Input: part model. Units: mm. Frame: model coordinates. A direction names the side the tool comes from. Give positions to 0.01 mm unless a question says otherwise; leave off trailing zeros. Write each loop counter-clockwise with the first axis right and the second up, starting at its lowest first coordinate (ties: lowest second). Pieces come first, ordered by that corner, then holes.
```python
from build123d import *

# Parameters (mm, degrees)
CROQUIS1_W              = 360
CROQUIS1_H              = 187
SALIENTE_EXTRUIR1_DEPTH = 80
VACIADO1_T              = -4
CORTAR_EXTRUIR1_DEPTH   = 361


with BuildPart() as part:
    # Croquis1 → Saliente-Extruir1 (new body)
    with BuildSketch(Plane(origin=(0, 0, 0), x_dir=(1, 0, 0), z_dir=(0, 1, 0))):
        Rectangle(CROQUIS1_W, CROQUIS1_H)
    extrude(amount=SALIENTE_EXTRUIR1_DEPTH)

    # Vaciado1
    vaciado1_openings = [part.faces().sort_by_distance(p)[0] for p in [
        (0, 80, 0),
    ]]
    offset(amount=VACIADO1_T, openings=vaciado1_openings, kind=Kind.INTERSECTION)

    # Croquis2 → Cortar-Extruir1 (cut, through all)
    with BuildSketch(Plane.ZY.offset(180)):
        Polygon((-93.5, 80), (93.5, 40), (93.5, 80), align=None)
    extrude(amount=-CORTAR_EXTRUIR1_DEPTH, mode=Mode.SUBTRACT)


solid = part.part
```
Item 1: Ray query, line 1 (X direction, y = 54, z = 12); line 2 (Z direction, x = 82, y = 24); line 3 (Y direction, x = -21, z = -2). Return the intervals inside material, ascending.
Item 2: Pin query (flat end, axial travel): pin 1 (10 mm diameter, centred on x = 22, z = 22, fed in from -Y); pin 2 (2 mm diameter, centred on x = 104.5, z = -65.5, fed in from +Y). Return the tip coordinate at first contact, or that it passes through.
Item 3: Section B-B (x = 78). Return loops of the section in (y, z), and give its area (3 significant figures).
Item 4: Section A-A (y = 34). Return loops of the section in (x, z).
Item 5: Mould query, pull axis Z, two halves, no side actions, for faces 1 (the flat face through (-0.84, 79.35, -90.47)), 2 (the flat face through (-2, 41, -89.5)), 3 (the flat face through (180, 31, 1)), 4 (the flat face through (-3, 39, -93.5)). Classes: +Z half, -Z half, draft (parallel to the pull), parting line (faces both ways), or undercut.
Item 6: Section C-C (y = 58). Return loops of the section in (x, z), and give its area (3 significant figures).
Item 7: Set-up query: faces 5 (the flat face through (176, 33, 1)), 6 (the flat face through (-180, 31, 1)). Return all of +Z, -Z, +X, -X, +Y, -Y with unobstructed straight access to the full face (end or side cutting, diameter ignored); none if empty.
Solved:
1. line 1: x = -180 to -176, 176 to 180
1. line 2: z = -93.5 to -89.5, 89.5 to 93.5
1. line 3: y = 0 to 4
2. pin 1: stops at y = 0
2. pin 2: stops at y = 4
3. outline: (0, -93.5) - (80, -93.5) - (79.14, -89.5) - (4, -89.5) - (4, 89.5) - (40.86, 89.5) - (40, 93.5) - (0, 93.5) - close
3. area: 1,200 mm2
4. outline: (-180, -93.5) - (180, -93.5) - (180, 93.5) - (-180, 93.5) - close; hole (-176, -89.5) - (176, -89.5) - (176, 89.5) - (-176, 89.5) - close
5. face 1: +Z half
5. face 2: undercut
5. face 3: draft
5. face 4: -Z half
6. outline: (-180, -93.5) - (180, -93.5) - (180, 9.35) - (176, 9.35) - (176, -89.5) - (-176, -89.5) - (-176, 9.35) - (-180, 9.35) - close
6. area: 2,230 mm2
7. face 5: +Y
7. face 6: +Z, -Z, -X, +Y, -Y
